Design review of the part shown in the three views and the two pictorial views. Dimensions are in mm from the part's minimum x, y and z. A direction names the side the tool comes from. Give positions to 0.01 mm unless a question says otherwise; leave off trailing zeros. Loops run counter-clockwise (first coordinate to the right, second up) from the corner with the lowest first, then second, coordinate; pieces in that order, holes last. Notation, with made-up numbers: (-19, 57) - (-15, 57) arc R25 cw to (-15, 81) - close; hole circle Ø4 at (12.25, 88.5). An arc over 180 degrees is marked (long way). Answer in a Markdown table with one row per item.
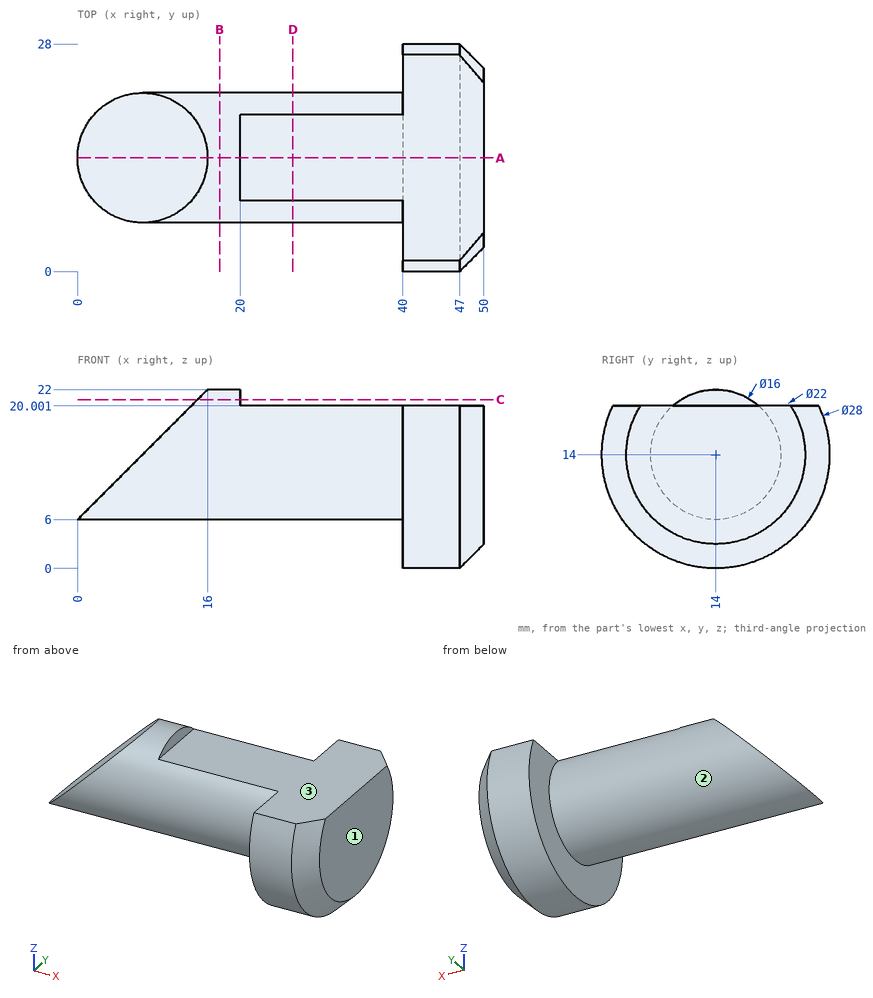
1. Clearance check with flat-ended pins moving along their axes: pin 1 (6 mm diameter, centred on x = 8.5, z = 9, fed in from -Y); pin 2 (12.5 mm diameter, centred on x = 35.5, y = 18.5, fed in from +Z); pin 3 (8 mm diameter, centred on x = 5.5, y = 18, fed in from -Z). State where each tip first meets the part, or that it passes through.
Values:
| item | result |
|---|---|
| pin 1 | stops at y = 6.25 |
| pin 2 | stops at z = 20 |
| pin 3 | stops at z = 6 |
2. We need section C-C, the plane z = 20.75. Give the boundary of the cut face in (x, y).
Values:
| item | result |
|---|---|
| outline | (14.75, 9.71) - (20, 9.71) - (20, 18.29) - (14.75, 18.29) - close |
3. For the marked faces 1, 2 and 3, list the 3-axis set-ups (+Z, -Z, +X, -X, +Y, -Y) from which the entire face can be reached by the end or side of a thin tool; tool diameter is ignored.
Values:
| item | result |
|---|---|
| face 1 | +Z, -Z, +X, +Y, -Y |
| face 2 | -X |
| face 3 | +Z, +X, +Y, -Y |
4. We need section B-B, the plane x = 17.5. Give the boundary of the cut face in (y, z).
Values:
| item | result |
|---|---|
| outline | circle Ø16 at (14, 14) |
5. We need section D-D, the plane x = 26.5. Give the boundary of the cut face in (y, z), and give its area (3 significant figures).
Values:
| item | result |
|---|---|
| outline | (8.71, 20) arc R8 ccw (long way) to (19.29, 20) - close |
| area | 187 mm^2 |
6. Wall thickness on line 1 (X direction, y = 24.5, z = 16.5); line 2 (Y direction, x = 27, z = 8); line 3 (X direction, y = 14.5, z = 12.5): over which ranges is each line inside the solid? List them lowest first. Write a range as [from, to].
Values:
| item | result |
|---|---|
| line 1 | x = [40, 50] |
| line 2 | y = [8.71, 19.29] |
| line 3 | x = [6.5, 50] |
7. We need section A-A, the plane y = 14. Give the boundary of the cut face in (x, z).
Values:
| item | result |
|---|---|
| outline | (0, 6) - (40, 6) - (40, 0) - (47, 0) - (50, 3) - (50, 20) - (20, 20) - (20, 22) - (16, 22) - close |
